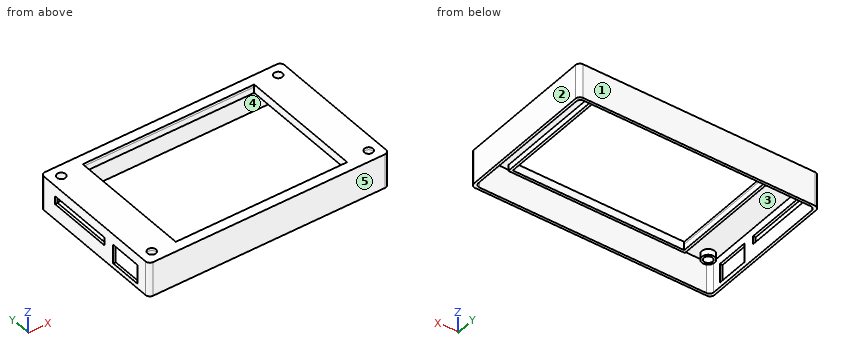
Autodesk Inventor part; units mm, degrees
ref_plane "Arbeitsebene1" through (-55, -32.5, -4) normal (0, 0, 1) x (1, 0, 0)
ref_plane "YZ Plane" through (0, 0, 0) normal (1, 0, 0) x (0, 1, 0)
ref_plane "XZ Plane" through (0, 0, 0) normal (0, 1, 0) x (-1, 0, 0)
sketch "Skizze1" plane through (0, 0, 0) normal (0, 0, 1) x (1, 0, 0)
  line L0 (-40.3, -29.3) -> (40.3, -29.3)
  line L1 (40.3, -29.3) -> (40.3, 29.3)
  line L2 (40.3, 29.3) -> (-40.3, 29.3)
  line L3 (-40.3, 29.3) -> (-40.3, -29.3)
  line L4 (40, 29) -> (-40, 29)
  line L5 (-40, 29) -> (-40, -29)
  line L6 (-40, -29) -> (40, -29)
  line L7 (40, -29) -> (40, 29)
  line L8 (-56.5, -34) -> (56.5, -34)
  line L9 (56.5, -34) -> (56.5, 34)
  line L10 (56.5, 34) -> (-56.5, 34)
  line L11 (-56.5, 34) -> (-56.5, -34)
  line L12 (53, 32.5) -> (-53, 32.5)
  line L13 (-53, -32.5) -> (53, -32.5)
  line L14 (55, -30.5) -> (55, 30.5)
  line L15 (-55, 30.5) -> (-55, -30.5)
  circle A0 centre (-51, 28.5) radius 2
  circle A1 centre (51, 28.5) radius 2
  circle A2 centre (51, -28.5) radius 2
  circle A3 centre (-51, -28.5) radius 2
  point P0 (0, 0)
  dimension "d0" = 0.3
  dimension "d1" = 0.3
  dimension "d2" = 0.3
  dimension "d3" = 0.3
  dimension "d4" = 1.5
  dimension "d5" = 1.5
  dimension "d6" = 1.5
  dimension "d7" = 1.5
extrude "Extrusion1" add sketch "Skizze1" against normal blind 1.2 contours L11 L10 L9 L8
sketch "Skizze2" plane through (0, 0, -1.2) normal (0, 0, -1) x (-1, 0, 0)
  circle A0 centre (-51, 28.5) radius 2
  circle A1 centre (51, 28.5) radius 2
  circle A2 centre (51, -28.5) radius 2
  circle A3 centre (-51, -28.5) radius 2
  circle A4 centre (-51, 28.5) radius 3
  circle A5 centre (51, 28.5) radius 3
  circle A6 centre (-51, -28.5) radius 3
  circle A7 centre (51, -28.5) radius 3
  line L0 (-40.3, -29.3) -> (-40.3, 29.3)
  line L1 (-40.3, 29.3) -> (40.3, 29.3)
  line L2 (-40.3, -29.3) -> (40.3, -29.3)
  line L3 (40.3, -29.3) -> (40.3, 29.3)
  line L4 (40.3, 29.3) -> (-40.3, 29.3)
  line L5 (-40.3, 29.3) -> (-40.3, -29.3)
  line L6 (41.5, 30.5) -> (-41.5, 30.5)
  line L7 (-41.5, 30.5) -> (-41.5, -30.5)
  line L8 (-41.5, -30.5) -> (41.5, -30.5)
  line L9 (41.5, -30.5) -> (41.5, 30.5)
  point P0 (0, 0)
  point P1 (53.2361, -26.5)
  point P2 (48.7639, -26.5)
  point P3 (51, -26.5)
  dimension "d10" = 6
  dimension "d11" = 6
  dimension "d12" = 6
  dimension "d13" = 6
  dimension "d14" = 1.2
  dimension "d15" = 1.2
  dimension "d16" = 1.2
  dimension "d17" = 1.2
ref_plane "Arbeitsebene1" through (-55, -32.5, -4) normal (0, 0, 1) x (1, 0, 0)
extrude "Extrusion2" add sketch "Skizze2" along normal up to surface (2.8 mm away)
sketch "Skizze3" plane through (0, 0, -1.2) normal (0, 0, -1) x (-1, 0, 0)
  line L0 (-56.5, -34) -> (56.5, -34)
  line L1 (-56.5, 34) -> (-56.5, -34)
  line L2 (56.5, -34) -> (-56.5, -34)
  line L3 (-56.5, -34) -> (-56.5, 34)
  line L4 (-56.5, 34) -> (56.5, 34)
  line L5 (56.5, 34) -> (56.5, -34)
  line L6 (-55.3, 32.8) -> (55.3, 32.8)
  line L7 (55.3, 32.8) -> (55.3, -32.8)
  line L8 (55.3, -32.8) -> (-55.3, -32.8)
  line L9 (-55.3, -32.8) -> (-55.3, 32.8)
  point P0 (0, 0)
  dimension "d20" = 1.2
  dimension "d21" = 1.2
  dimension "d22" = 1.2
  dimension "d23" = 1.2
extrude "Extrusion3" add sketch "Skizze3" along normal blind 15
fillet "Rundung1" radius 2 8 edges at (55.3, 32.8, -8.7) (-55.3, 32.8, -8.7) (-55.3, -32.8, -8.7) (56.5, -34, -8.1) (-56.5, -34, -8.1) (-56.5, 34, -8.1) (56.5, 34, -8.1) (55.3, -32.8, -8.7)
sketch "Skizze4" plane through (-56.5, -32, 0) normal (-1, 0, 0) x (0, 0, 1)
  line L0 (-5.5, 1.5) -> (-5.5, 5.5) construction
  line L1 (-5.5, 1.5) -> (-4, 1.5) construction
  line L2 (-4, 62.5) -> (-4, 1.5) construction
  line L3 (-5.5, 62.5) -> (-4, 62.5) construction
  line L4 (-5.5, 56.5) -> (-5.5, 62.5) construction
  line L5 (-5.5, 56.5) -> (-8.3, 56.5) construction
  line L6 (-8.3, 26.5) -> (-8.3, 56.5) construction
  line L7 (-5.5, 26.5) -> (-8.3, 26.5) construction
  line L8 (-5.5, 20) -> (-5.5, 26.5) construction
  line L9 (-5.5, 20) -> (-13.5, 20) construction
  line L10 (-13.5, 5.5) -> (-13.5, 20) construction
  line L11 (-5.5, 5.5) -> (-13.5, 5.5) construction
  line L12 (-5, 20.5) -> (-14, 20.5)
  line L13 (-14, 20.5) -> (-14, 5)
  line L14 (-14, 5) -> (-5, 5)
  line L15 (-5, 5) -> (-5, 20.5)
  line L16 (-5, 26) -> (-8.8, 26)
  line L17 (-8.8, 26) -> (-8.8, 57)
  line L18 (-8.8, 57) -> (-5, 57)
  line L19 (-5, 57) -> (-5, 26)
  point P0 (0, 32)
  dimension "d27" = 0.5
  dimension "d28" = 0.5
  dimension "d29" = 0.5
  dimension "d30" = 0.5
  dimension "d31" = 0.5
  dimension "d32" = 0.5
  dimension "d33" = 0.5
extrude "Extrusion4" cut sketch "Skizze4" against normal up to next
properties part number "front_case" material "ABS-Kunststoff"
Could you check a few things on this model? Use its own coordinates, in mm. Face numbers are marked on the shaded views. A direction names the side the tool comes from. Coordinates: 2 decimals unless noted, no trailing zeros. Loops run counter-clockwise (first coordinate to the right, second up) from the corner with the lowest first, then second, coordinate; pieces in that order, holes last.
1) Imagine slicing it at A-A (y = 17). List the corners of the cut face in (x, z) for me.
Reported:
outline: (-56.5, -16.2) - (-55.3, -16.2) - (-55.3, -8.8) - (-56.5, -8.8) - close; (-56.5, -5) - (-55.3, -5) - (-55.3, -1.2) - (-41.5, -1.2) - (-41.5, -4) - (-40.3, -4) - (-40.3, 0) - (-56.5, 0) - close; (40.3, -4) - (41.5, -4) - (41.5, -1.2) - (55.3, -1.2) - (55.3, -16.2) - (56.5, -16.2) - (56.5, 0) - (40.3, 0) - close
2) Which directions (+Z, -Z, +X, -X, +Y, -Y) give clear straight access to the entire face, cutting with the end or side of a thin tool? Please do the marked faces 4 and 5.
Reported:
face 4: -Z
face 5: +Z, -Z, +X, -X, -Y
3) Please list where these lines run through material, in increasing order: line 1 along Y through (x, z) = (51, -0.9); line 2 along Y through (x, z) = (-51, -1.85); line 3 along X through (y, z) = (23, -3.75).
Reported:
line 1: y = -34 to -30.5, -26.5 to 26.5, 30.5 to 34
line 2: y = -34 to -32.8, -31.5 to -30.5, -26.5 to -25.5, 25.5 to 26.5, 30.5 to 31.5, 32.8 to 34
line 3: x = -56.5 to -55.3, -41.5 to -40.3, 40.3 to 41.5, 55.3 to 56.5
4) Imagine slicing it at D-D (z = -10). List the corners of the cut face in (x, y) for me, and give its area (3 significant figures).
Reported:
outline: (-56.5, -32) arc R2 ccw to (-54.5, -34) - (54.5, -34) arc R2 ccw to (56.5, -32) - (56.5, 32) arc R2 ccw to (54.5, 34) - (-54.5, 34) arc R2 ccw to (-56.5, 32) - (-56.5, -11.5) - (-55.3, -11.5) - (-55.3, 30.8) arc R2 cw to (-53.3, 32.8) - (53.3, 32.8) arc R2 cw to (55.3, 30.8) - (55.3, -30.8) arc R2 cw to (53.3, -32.8) - (-53.3, -32.8) arc R2 cw to (-55.3, -30.8) - (-55.3, -27) - (-56.5, -27) - close
area: 410 mm2
5) Imagine slicing it at C-C (x = 31.5). List the corners of the cut face in (y, z) for me.
Reported:
outline: (-34, -16.2) - (-32.8, -16.2) - (-32.8, -1.2) - (-30.5, -1.2) - (-30.5, -4) - (-29.3, -4) - (-29.3, 0) - (-34, 0) - close; (29.3, -4) - (30.5, -4) - (30.5, -1.2) - (32.8, -1.2) - (32.8, -16.2) - (34, -16.2) - (34, 0) - (29.3, 0) - close
6) Imagine slicing it at B-B (x = -51). List the corners of the cut face in (y, z) for me, and give its area (3 significant figures).
Reported:
outline: (-34, -16.2) - (-32.8, -16.2) - (-32.8, -1.2) - (-31.5, -1.2) - (-31.5, -4) - (-30.5, -4) - (-30.5, 0) - (-34, 0) - close; (-26.5, -4) - (-25.5, -4) - (-25.5, -1.2) - (25.5, -1.2) - (25.5, -4) - (26.5, -4) - (26.5, 0) - (-26.5, 0) - close; (30.5, -4) - (31.5, -4) - (31.5, -1.2) - (32.8, -1.2) - (32.8, -16.2) - (34, -16.2) - (34, 0) - (30.5, 0) - close
area: 119 mm2
7) Will these pins go through, and if not, where does the flat tip stop? pin 1 Ø1.3 at (x, z) = (-55.5, -7.5) entering from +Y; pin 2 Ø4.5 at (x, y) = (-51, -28.5) entering from -Z; pin 3 Ø3 at (x, y) = (44.5, 26.5) entering from -Z.
Reported:
pin 1: stops at y = 33.97
pin 2: stops at z = -4
pin 3: stops at z = -1.2
8) Thinking about a two-plate mould opening in X: for the marked faces 1, 2 and 3, which applies, released by +X, released by -X, zero draft, split by the parting line, or undercut?
Reported:
face 1: zero draft
face 2: released by +X
face 3: undercut
